Read the model definition and answer for the solid it produces. Units are mm, in the model's axes. Give positions to 0.01 mm unless a question says otherwise; leave off trailing zeros. Loops run counter-clockwise (first coordinate to the right, second up) from the corner with the lowest first, then second, coordinate; pieces in that order, holes last. Notation, with made-up numbers: (-1, 12) -> (20, 12) arc R7 ccw to (20, 25) -> close; hole circle Ø11 at (46, 80). An arc over 180 degrees is marked (long way). Return JSON: item names as keys, results as strings. Group by question number.
Autodesk Inventor part; units mm, degrees
ref_plane "YZ Plane" through (0, 0, 0) normal (1, 0, 0) x (0, 1, 0)
ref_plane "XZ Plane" through (0, 0, 0) normal (0, 1, 0) x (-1, 0, 0)
ref_plane "XY Plane" through (0, 0, 0) normal (0, 0, 1) x (1, 0, 0)
sketch "スケッチ1" plane through (0, 0, 0) normal (0, 1, 0) x (-1, 0, 0)
  circle A0 centre (0, 0) radius 10
  circle A1 centre (0, 0) radius 5
  dimension "d0" = 20
  dimension "d2" = 10
extrude "押し出し1" add sketch "スケッチ1" along normal blind 1
sketch "スケッチ2" plane through (0, 1, 0) normal (0, 1, 0) x (1, 0, 0)
  circle A0 centre (0, 0) radius 5
  circle A1 centre (0, 7) radius 1
  dimension "d5" = 2
  dimension "d7" = 7
  dimension "d8" = 0
hole "穴1" at (0, 1, -7) direction (0, -1, 0) diameter 2 end through all
pattern_circular "円形状パターン1" count 8 over 360 about axis through (0, 0, 0) along (0, 1, 0) of "穴1"
properties part number "8" material "アセタール樹脂、白"
1. Determine the mould class of faces 1 (the cylindrical face through (1.08, 0.49, 4.88)), 2 (the cylindrical face through (2.17, 0.49, 9.76)), 3 (the flat face through (-2, 1, 5)) for opening direction Z: pulls with the +Z half, pulls with the -Z half, needs draft (parallel to the pull), parting line crosses it, or undercut.
2. Section B-B on x = 0 is taken. Determine the outline of the cut face in (y, z).
3. Flat-ended cylindrical pins translate along their axes: pin 1 Ø1.8 at (x, z) = (0, -7) entering from -Y; pin 2 Ø5 at (x, z) = (-0.5, -2.5) entering from +Y. Find the tip coordinate at first contact, or state that the pin passes through.
4. Section C-C on z = -7 is taken. Determine the outline of the cut face in (x, y), then the cut area to 3 significant figures.
5. Straight lines are drawn through the part: line 1 (Z direction, x = 4.5, y = 0.25); line 2 (X direction, y = 0.5, z = 5.75); line 3 (X direction, y = 0.3, z = 5.5). For each, find the intervals that lie inside material, in ascending order. Write a range as from..to.
6. Section D-D on x = 2.5 is taken. Determine the outline of the cut face in (y, z), then the cut area to 3 significant figures.
7. Section A-A on z = 0 is taken. Determine the outline of the cut face in (x, y).
Completed:
{
 "1": {"face 1": "undercut", "face 2": "parting line crosses it", "face 3": "needs draft"},
 "2": {"outline": "(0, -10) -> (1, -10) -> (1, -8) -> (0, -8) -> close; (0, -6) -> (1, -6) -> (1, -5) -> (0, -5) -> close; (0, 5) -> (1, 5) -> (1, 6) -> (0, 6) -> close; (0, 8) -> (1, 8) -> (1, 10) -> (0, 10) -> close"},
 "3": {"pin 1": "passes through", "pin 2": "stops at y = 1"},
 "4": {"outline": "(-7.14, 0) -> (-1, 0) -> (-1, 1) -> (-7.14, 1) -> close; (1, 0) -> (7.14, 0) -> (7.14, 1) -> (1, 1) -> close", "area": "12.3 mm²"},
 "5": {"line 1": "z = -8.93..-5.84, -4.06..-2.18, 2.18..4.06, 5.84..8.93", "line 2": "x = -8.18..-5.55, -4.35..4.35, 5.55..8.18", "line 3": "x = -8.35..-5.78, -4.11..4.11, 5.78..8.35"},
 "6": {"outline": "(0, -9.68) -> (1, -9.68) -> (1, -4.33) -> (0, -4.33) -> close; (0, 4.33) -> (1, 4.33) -> (1, 9.68) -> (0, 9.68) -> close", "area": "10.7 mm²"},
 "7": {"outline": "(-10, 0) -> (-8, 0) -> (-8, 1) -> (-10, 1) -> close; (-6, 0) -> (-5, 0) -> (-5, 1) -> (-6, 1) -> close; (5, 0) -> (6, 0) -> (6, 1) -> (5, 1) -> close; (8, 0) -> (10, 0) -> (10, 1) -> (8, 1) -> close"}
}
